CAD build for the part. Positions are in the model's coordinates, mm. Face numbers are marked on the shaded views. A direction names the side the tool comes from. Round coordinates to 2 decimals unless told otherwise and drop trailing zeros. Order: outer loops, then holes, each group sorted by start corner. A loop starts at its lowest first (then second) coordinate and runs counter-clockwise, first axis right, second up. Notation, with made-up numbers: M -25,-37 L 34,-37 A16 cw 34,-18 Z; hole C 9.5,10.25 d5. An arc over 180 degrees is marked long. Answer as CSV lines item,"result". Start each with the question number.
```python
from build123d import *

# Parameters (mm, degrees)
SKETCH1_W           = 50
SKETCH1_H           = 50
BOSS_EXTRUDE1_DEPTH = 25
SKETCH2_R           = 8
CUT_EXTRUDE1_DEPTH  = 58
SKETCH3_R           = 3
CUT_EXTRUDE2_DEPTH  = 25
SKETCH4_W           = 63
SKETCH4_H           = 15
BOSS_EXTRUDE2_DEPTH = 6
SKETCH5_R           = 2
CUT_EXTRUDE3_DEPTH  = 6
CHAMFER1_SIZE       = 2.5
FILLET1_R           = 3


with BuildPart() as part:
    # Sketch1 → Boss-Extrude1 (new body)
    with BuildSketch(Plane.XY):
        with Locations((25, 25)):
            Rectangle(SKETCH1_W, SKETCH1_H)
    extrude(amount=BOSS_EXTRUDE1_DEPTH)

    # Sketch2 → Cut-Extrude1 (cut)
    with BuildSketch(Plane.ZY):
        with Locations((25, 25)):
            Circle(SKETCH2_R)
    extrude(amount=-CUT_EXTRUDE1_DEPTH, mode=Mode.SUBTRACT)

    # Sketch3 → Cut-Extrude2 (cut)
    with BuildSketch(Plane.XY.offset(25)):
        with Locations((15, 40)):
            Circle(SKETCH3_R)
        with Locations((35, 40)):
            Circle(SKETCH3_R)
        with Locations((35, 10)):
            Circle(SKETCH3_R)
        with Locations((15, 10)):
            Circle(SKETCH3_R)
    extrude(amount=-CUT_EXTRUDE2_DEPTH, mode=Mode.SUBTRACT)

    # Sketch4 → Boss-Extrude2 (add)
    with BuildSketch(Plane.ZY):
        with Locations((31.5, 42.5)):
            Rectangle(SKETCH4_W, SKETCH4_H)
        with Locations((31.5, 7.5)):
            Rectangle(SKETCH4_W, SKETCH4_H)
    extrude(amount=BOSS_EXTRUDE2_DEPTH)

    # Sketch5 → Cut-Extrude3 (cut)
    with BuildSketch(Plane.ZY.offset(6)):
        with Locations((54, 42.5)):
            Circle(SKETCH5_R)
        with Locations((54, 7.5)):
            Circle(SKETCH5_R)
    extrude(amount=-CUT_EXTRUDE3_DEPTH, mode=Mode.SUBTRACT)

    # Chamfer1
    chamfer1_edges = [part.edges().sort_by_distance(p)[0] for p in [
        (-6, 42.5, 52),
        (-6, 7.5, 52),
    ]]
    chamfer(chamfer1_edges, length=CHAMFER1_SIZE)

    # Fillet1
    # the kernel refuses this fillet: 3 mm, written as the material it adds along each edge
    with BuildSketch(Plane(origin=(0, 15, 25), x_dir=(-1, 0, 0), z_dir=(0, 0, -1))) as fillet1_piece_1_section:
        with BuildLine():
            CenterArc((FILLET1_R, FILLET1_R), FILLET1_R, 180, 90)
            Line((0, FILLET1_R), (0, 0))
            Line((0, 0), (FILLET1_R, 0))
        make_face()
    fillet1_piece_1 = extrude(amount=25, mode=Mode.PRIVATE)
    fillet1_piece_1 = fillet1_piece_1 - Plane(origin=(-0.671433756, 25, 25), x_dir=(0, 0, 1), z_dir=(-1, 0, 0)) * Cylinder(8, 62, mode=Mode.PRIVATE)
    add(fillet1_piece_1)
    with BuildSketch(Plane(origin=(0, 35, 25), x_dir=(-1, 0, 0), z_dir=(0, 0, -1))) as fillet1_piece_2_section:
        with BuildLine():
            CenterArc((FILLET1_R, -FILLET1_R), FILLET1_R, 90, 90)
            Line((0, -FILLET1_R), (0, 0))
            Line((0, 0), (FILLET1_R, 0))
        make_face()
    fillet1_piece_2 = extrude(amount=25, mode=Mode.PRIVATE)
    fillet1_piece_2 = fillet1_piece_2 - Plane(origin=(-0.671433756, 25, 25), x_dir=(0, 0, 1), z_dir=(-1, 0, 0)) * Cylinder(8, 62, mode=Mode.PRIVATE)
    add(fillet1_piece_2)


solid = part.part
```
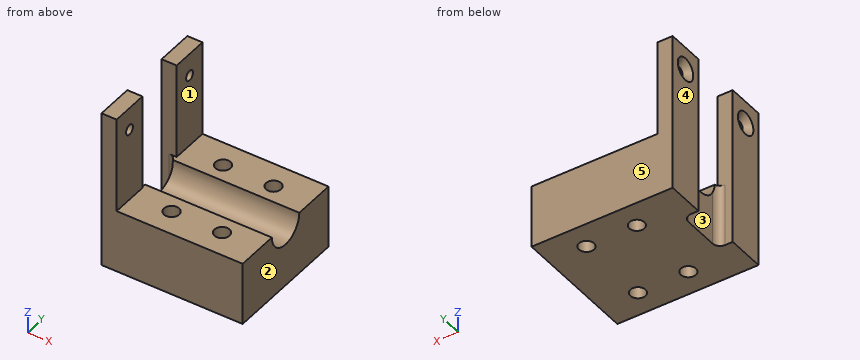
Q1. Band-saw the part on A-A, the plane x = 15. Write the cut outline in (y, z).
Q2. Mould opens along Y. For the marked faces 3, 4 and 5 say: +Y half, -Y half, draft (parallel to the pull), parting line (faces both ways), or undercut.
Q3. Band-saw the part on C-C, the plane z = 14. Write the cut outline in (x, y), then the cut area to 3 significant figures.
Q4. Tool access for the marked faces 1 and 2: list every direction of +Z, -Z, +X, -X, +Y, -Y with a clear straight run to the whole face (end or side of a thin tool).
Q5. Probe line 1 along Y through (x, z) = (15, 6); line 2 along Y through (x, z) = (-2, 54); line 3 along Y through (x, z) = (35, 19). List the from-to ranges inside material, lowest first. Write a range as from..to.
Q6. Band-saw the part on D-D, the plane x = 8.5. Write the cut outline in (y, z), then the cut area to 3 significant figures.
Q7. Band-saw the part on B-B, the plane z = 47.5. Write the cut outline in (x, y).
Q8. Drop flat-ended pins along their axis: P1, Ø5, axis at x = 7.5, y = 38, coming from the -Z side; P2, Ø12, axis at x = 41.5, y = 17, coming from the +Z side; P3, Ø8, axis at y = 13.5, z = 51.5, coming from the +X side; P4, Ø3.5, axis at x = 15, y = 10, coming from the +Z side. Give the stop position or say it passes through.
Answer:
1,outline,"M 0,0 L 7,0 L 7,25 L 0,25 Z; M 13,0 L 37,0 L 37,25 L 33,25 A8 cw 17,25 L 13,25 Z; M 43,0 L 50,0 L 50,25 L 43,25 Z"
2,face 3,"undercut"
2,face 4,"draft"
2,face 5,"+Y half"
3,outline,"M -6,0 L 50,0 L 50,50 L -6,50 L -6,35 L -3,35 A3 cw 0,32 L 0,18 A3 cw -3,15 L -6,15 Z; hole C 15,10 d6; hole C 15,40 d6; hole C 35,10 d6; hole C 35,40 d6"
3,area,"2,570 mm^2"
4,face 1,"+Z, +X, +Y, -Y"
4,face 2,"+Z, -Z, +X, +Y, -Y"
5,line 1,"y = 0..7, 13..37, 43..50"
5,line 2,"y = 0..5.5, 9.5..15, 35..40.5, 44.5..50"
5,line 3,"y = 0..7, 13..19.71, 30.29..37, 43..50"
6,outline,"M 0,0 L 50,0 L 50,25 L 33,25 A8 cw 17,25 L 0,25 Z"
6,area,"1,150 mm^2"
7,outline,"M -6,0 L 0,0 L 0,15 L -6,15 Z; M -6,35 L 0,35 L 0,50 L -6,50 Z"
8,P1,"stops at z = 0"
8,P2,"stops at z = 25"
8,P3,"stops at x = 0"
8,P4,"passes through"
